For this review, take the finished solid that the model builds, in its own axes (mm). A direction names the side the tool comes from. Give positions to 0.01 mm unless a question says otherwise; leave off trailing zeros. Loops run counter-clockwise (first coordinate to the right, second up) from the corner with the lowest first, then second, coordinate; pieces in that order, holes last. Notation, with made-up numbers: (-5, 62) - (36, 62) arc R6 ccw to (36, 66) - close; hole circle Ø5 at (24, -22.75). An arc over 180 degrees is marked (long way). Answer as CSV lines item,"result".
from build123d import *

# Parameters (mm, degrees)
SALIENTE_EXTRUIR1_DEPTH = 4
CROQUIS2_W              = 55
CROQUIS2_H              = 61
CORTAR_EXTRUIR1_DEPTH   = 2
CROQUIS4_W              = 7
CROQUIS4_H              = 2
CORTAR_EXTRUIR2_DEPTH   = 9
CROQUIS6_W              = 7
CROQUIS6_H              = 2
CORTAR_EXTRUIR3_DEPTH   = 9
CROQUIS7_W              = 7
CROQUIS7_H              = 2
CORTAR_EXTRUIR4_DEPTH   = 9
CROQUIS8_W              = 7
CROQUIS8_H              = 2
CORTAR_EXTRUIR5_DEPTH   = 9


with BuildPart() as part:
    # Croquis1 → Saliente-Extruir1 (new body)
    with BuildSketch(Plane(origin=(0, 0, 0), x_dir=(1, 0, 0), z_dir=(0, 1, 0))):
        Polygon((30, -32.5), (30, -22.5), (41, -22.5), (41, -11.5), (30, -11.5), (30, 11.5), (41, 11.5), (41, 22.5), (30, 22.5), (30, 32.5), (-30, 32.5), (-30, 22.5), (-41, 22.5), (-41, 11.5), (-30, 11.5), (-30, -11.5), (-41, -11.5), (-41, -22.5), (-30, -22.5), (-30, -32.5), align=None)
    extrude(amount=SALIENTE_EXTRUIR1_DEPTH)

    # Croquis2 → Cortar-Extruir1 (cut)
    with BuildSketch(Plane(origin=(0, 4, 0), x_dir=(1, 0, 0), z_dir=(0, 1, 0))):
        Rectangle(CROQUIS2_W, CROQUIS2_H)
    extrude(amount=-CORTAR_EXTRUIR1_DEPTH, mode=Mode.SUBTRACT)

    # Croquis4 → Cortar-Extruir2 (cut)
    with BuildSketch(Plane.ZY.offset(41)):
        with Locations((-17, 2)):
            Rectangle(CROQUIS4_W, CROQUIS4_H)
    extrude(amount=-CORTAR_EXTRUIR2_DEPTH, mode=Mode.SUBTRACT)

    # Croquis6 → Cortar-Extruir3 (cut)
    with BuildSketch(Plane.ZY.offset(41)):
        with Locations((17, 2)):
            Rectangle(CROQUIS6_W, CROQUIS6_H)
    extrude(amount=-CORTAR_EXTRUIR3_DEPTH, mode=Mode.SUBTRACT)

    # Croquis7 → Cortar-Extruir4 (cut)
    with BuildSketch(Plane(origin=(41, 0, 0), x_dir=(0, 0, -1), z_dir=(1, 0, 0))):
        with Locations((-17, 2)):
            Rectangle(CROQUIS7_W, CROQUIS7_H)
    extrude(amount=-CORTAR_EXTRUIR4_DEPTH, mode=Mode.SUBTRACT)

    # Croquis8 → Cortar-Extruir5 (cut)
    with BuildSketch(Plane(origin=(41, 0, 0), x_dir=(0, 0, -1), z_dir=(1, 0, 0))):
        with Locations((17, 2)):
            Rectangle(CROQUIS8_W, CROQUIS8_H)
    extrude(amount=-CORTAR_EXTRUIR5_DEPTH, mode=Mode.SUBTRACT)


solid = part.part
1) Insertion check: P1, Ø1.6, axis at y = 2, z = 17.5, coming from the -X side; P2, Ø1.2, axis at y = 1, z = 29.5, coming from the +X side; P3, Ø1.6, axis at x = 38, y = 2.5, coming from the -Z side. Each pin has a flat end and moves straight along its axis. Give the tip position at first contact, or say it passes through.
From the geometry:
P1,"stops at x = -32"
P2,"stops at x = 30"
P3,"stops at z = -22.5"
2) Consider section C-C on z = 18.5. Write out the cut boundary in (x, y), and give its area (3 significant figures).
From the geometry:
outline,"(-41, 0) - (41, 0) - (41, 1) - (32, 1) - (32, 3) - (41, 3) - (41, 4) - (27.5, 4) - (27.5, 2) - (-27.5, 2) - (-27.5, 4) - (-41, 4) - (-41, 3) - (-32, 3) - (-32, 1) - (-41, 1) - close"
area,"182 mm^2"
3) Draft analysis for pull direction Y (two halves, no side actions). For faces 4 (the flat face through (-1, 0, 0)), 5 (the flat face through (-32, 2, 17)), 6 (the flat face through (-27.5, 3, 0)), state which applies: pulls with the +Y half, pulls with the -Y half, needs draft (parallel to the pull), parting line crosses it, or undercut.
From the geometry:
face 4,"pulls with the -Y half"
face 5,"undercut"
face 6,"needs draft"
4) Wall thickness on line 1 (Z direction, x = -34, y = 2.3); line 2 (Z direction, x = 23, y = 2.1); line 3 (X direction, y = 3.2, z = 9): over which ranges is each line inside the solid? List them lowest first. Write a range as from..to.
From the geometry:
line 1,"z = -22.5..-20.5, -13.5..-11.5, 11.5..13.5, 20.5..22.5"
line 2,"z = -32.5..-30.5, 30.5..32.5"
line 3,"x = -30..-27.5, 27.5..30"
5) Consider section A-A on z = 9.5. Write out the cut boundary in (x, y), and give its area (3 significant figures).
From the geometry:
outline,"(-30, 0) - (30, 0) - (30, 4) - (27.5, 4) - (27.5, 2) - (-27.5, 2) - (-27.5, 4) - (-30, 4) - close"
area,"130 mm^2"
6) Consider section B-B on x = 12. Write out the cut boundary in (y, z).
From the geometry:
outline,"(0, -32.5) - (4, -32.5) - (4, -30.5) - (2, -30.5) - (2, 30.5) - (4, 30.5) - (4, 32.5) - (0, 32.5) - close"
7) Machinability: for faces 1 (the flat face through (30, 2, 28)), 2 (the flat face through (37, 2, -20.5)), 3 (the flat face through (36, 2, -22.5)), which of the approach directions +Z, -Z, +X, -X, +Y, -Y give a long, thin tool a straight path to every point of the face, cutting with its end or side? Answer none if there is none.
From the geometry:
face 1,"+Z, +X, +Y, -Y"
face 2,"+X"
face 3,"-Z, +X, +Y, -Y"
